Verification items for the finished model (mm, model axes). Face numbers are marked on the shaded views. A direction names the side the tool comes from. Coordinates: 2 decimals unless noted, no trailing zeros. Order: outer loops, then holes, each group sorted by start corner. A loop starts at its lowest first (then second) coordinate and runs counter-clockwise, first axis right, second up. Notation, with made-up numbers: M 69,-32.5 L 100,-32.5 A13 cw 100,-12.5 Z; hole C -3.75,-3 d10. An arc over 180 degrees is marked long. Return JSON: item names as keys, results as strings. Group by question number.
1. Material ranges on line 1 along Y through (x, z) = (-51.75, 5); line 2 along Y through (x, z) = (-42.5, 4.5); line 3 along X through (y, z) = (-14, 4), recorded low to high.
2. Section check D-D, the plane z = 1. Record the cut outline in (x, y).
3. Section check B-B, the plane x = -46.5. Record the cut outline in (y, z), plus the area to 3 significant figures.
4. Set-up check for the marked faces 4 and 5: record each of +Z, -Z, +X, -X, +Y, -Y from which the full face is reachable in a straight line by a thin tool's end or side.
5. Mould release check, pull along X, two halves, no side actions. Record for the marked faces 1, 2 and 3: +X half, -X half, draft (parallel to the pull), parting line (faces both ways), or undercut.
6. Section check A-A, the plane y = -18. Record the cut outline in (x, z).
7. Gauge pin test, flat ends, axial feed: pin 1 (0.8 mm diameter, centred on x = -63.5, z = 4, fed in from -Y); pin 2 (2.5 mm diameter, centred on y = 13.89, z = 5, fed in from -X); pin 3 (2.5 mm diameter, centred on x = -69.5, z = 6, fed in from +Y). Record the tip position at first contact, or that the pin passes through.
8. Section check C-C, the plane y = 17. Record the cut outline in (x, z).
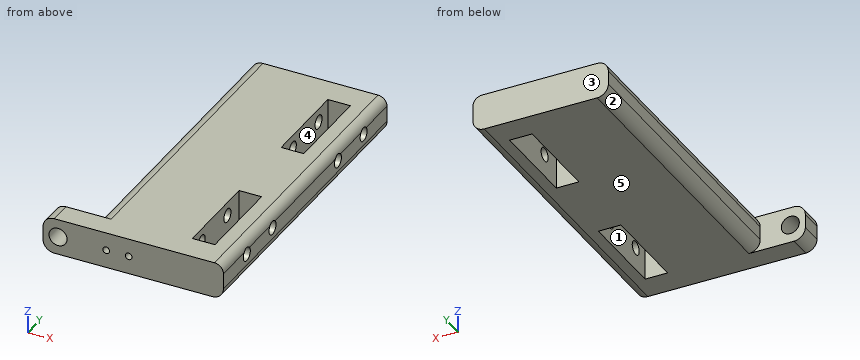
```python
from build123d import *

# Parameters (mm, degrees)
ESBO_O2_W                = 30
ESBO_O2_H                = 70
RESSALTO_EXTRUS_O1_DEPTH = 8
ESBO_O3_R                = 0.75
CORTE_EXTRUS_O1_DEPTH    = 30
FILETE1_R                = 2
ESBO_O17_W               = 10
ESBO_O17_H               = 5
RESSALTO_EXTRUS_O4_DEPTH = 8
ESBO_O20_R               = 2
CORTE_EXTRUS_O9_DEPTH    = 8
FILETE2_R                = 2.5
FILETE3_R                = 2.5
FILETE4_R                = 2.5
FILETE5_R                = 2.5
ESBO_O21_W               = 5
ESBO_O21_H               = 20
CORTE_EXTRUS_O10_DEPTH   = 9
FILETE6_R                = 2.5
ESBO_O22_R               = 1.5
CORTE_EXTRUS_O11_DEPTH   = 20


with BuildPart() as part:
    # Esboço2 → Ressalto-extrusão1 (new body)
    with BuildSketch(Plane.XY):
        with Locations((-52.281248797, -0.107598663)):
            Rectangle(ESBO_O2_W, ESBO_O2_H)
    extrude(amount=RESSALTO_EXTRUS_O1_DEPTH)

    # Esboço3 → Corte-extrusão1 (cut)
    with BuildSketch(Plane(origin=(0, -35.107598663, 0), x_dir=(-1, 0, 0), z_dir=(0, -1, 0))):
        with Locations((58.281248797, -4)):
            Circle(ESBO_O3_R)
        with Locations((63.281248797, -4)):
            Circle(ESBO_O3_R)
    extrude(amount=-CORTE_EXTRUS_O1_DEPTH, mode=Mode.SUBTRACT)

    # Filete1
    filete1_edges = [part.edges().sort_by_distance(p)[0] for p in [
        (-37.281248797, -0.107598663, 8),
    ]]
    fillet(filete1_edges, radius=FILETE1_R)

    # Esboço17 → Ressalto-extrusão4 (add)
    with BuildSketch(Plane(origin=(0, 0, 0), x_dir=(-1, 0, 0), z_dir=(0, 0, -1))):
        with Locations((72.281248797, -32.607598663)):
            Rectangle(ESBO_O17_W, ESBO_O17_H)
    extrude(amount=-RESSALTO_EXTRUS_O4_DEPTH)

    # Esboço20 → Corte-extrusão9 (cut)
    with BuildSketch(Plane.XZ.offset(35.107598663)):
        with Locations((-73.951248797, 4)):
            Circle(ESBO_O20_R)
    extrude(amount=-CORTE_EXTRUS_O9_DEPTH, mode=Mode.SUBTRACT)

    # Filete2
    filete2_edges = [part.edges().sort_by_distance(p)[0] for p in [
        (-67.281248797, 2.392401337, 8),
    ]]
    fillet(filete2_edges, radius=FILETE2_R)

    # Filete3
    filete3_edges = [part.edges().sort_by_distance(p)[0] for p in [
        (-67.281248797, 2.392401337, 0),
    ]]
    fillet(filete3_edges, radius=FILETE3_R)

    # Filete4
    filete4_edges = [part.edges().sort_by_distance(p)[0] for p in [
        (-77.281248797, -32.607598663, 8),
    ]]
    fillet(filete4_edges, radius=FILETE4_R)

    # Filete5
    filete5_edges = [part.edges().sort_by_distance(p)[0] for p in [
        (-77.281248797, -32.607598663, 0),
    ]]
    fillet(filete5_edges, radius=FILETE5_R)

    # Esboço21 → Corte-extrusão10 (cut, through all)
    with BuildSketch(Plane.XY.offset(8)):
        with Locations((-44.781248797, 18.892401337)):
            Rectangle(ESBO_O21_W, ESBO_O21_H)
        with Locations((-44.781248797, -19.107598663)):
            Rectangle(ESBO_O21_W, ESBO_O21_H)
    extrude(amount=-CORTE_EXTRUS_O10_DEPTH, mode=Mode.SUBTRACT)

    # Filete6
    filete6_edges = [part.edges().sort_by_distance(p)[0] for p in [
        (-37.281248797, -0.107598663, 0),
    ]]
    fillet(filete6_edges, radius=FILETE6_R)

    # Esboço22 → Corte-extrusão11 (cut)
    with BuildSketch(Plane(origin=(-37.281248797, 0, 0), x_dir=(0, 0, -1), z_dir=(1, 0, 0))):
        with Locations((-5, -25.107598663)):
            Circle(ESBO_O22_R)
        with Locations((-5, -14.107598663)):
            Circle(ESBO_O22_R)
        with Locations((-5, 24.892401337)):
            Circle(ESBO_O22_R)
        with Locations((-5, 13.892401337)):
            Circle(ESBO_O22_R)
    extrude(amount=-CORTE_EXTRUS_O11_DEPTH, mode=Mode.SUBTRACT)


solid = part.part
```
Answers follow:
{
 "1": {"line 1": "-35.11 to -26.61, -23.61 to -15.61, -12.61 to 12.39, 15.39 to 23.39, 26.39 to 34.89", "line 2": "-35.11 to -29.11, -9.11 to 8.89, 28.89 to 34.89", "line 3": "-67.28 to -64.03, -62.53 to -59.03, -57.53 to -57.28"},
 "2": {"outline": "M -76.78,-35.11 L -37.78,-35.11 L -37.78,34.89 L -66.78,34.89 L -66.78,-30.11 L -76.78,-30.11 Z; hole M -47.28,-29.11 L -42.28,-29.11 L -42.28,-9.11 L -47.28,-9.11 Z; hole M -47.28,8.89 L -42.28,8.89 L -42.28,28.89 L -47.28,28.89 Z"},
 "3": {"outline": "M -35.11,0 L -29.11,0 L -29.11,8 L -35.11,8 Z; M -9.11,0 L 8.89,0 L 8.89,8 L -9.11,8 Z; M 28.89,0 L 34.89,0 L 34.89,8 L 28.89,8 Z", "area": "240 mm^2"},
 "4": {"face 4": "+Z, -Z", "face 5": "-Z, +X, -X, +Y, -Y"},
 "5": {"face 1": "undercut", "face 2": "-X half", "face 3": "draft"},
 "6": {"outline": "M -67.28,2.5 A2.5 ccw -64.78,0 L -47.28,0 L -47.28,8 L -64.78,8 A2.5 ccw -67.28,5.5 Z; M -42.28,0 L -39.78,0 A2.5 ccw -37.28,2.5 L -37.28,6 A2 ccw -39.28,8 L -42.28,8 Z; hole C -63.28,4 d1.5; hole C -58.28,4 d1.5"},
 "7": {"pin 1": "y = -5.11", "pin 2": "x = -67.28", "pin 3": "y = -30.11"},
 "8": {"outline": "M -67.28,2.5 A2.5 ccw -64.78,0 L -47.28,0 L -47.28,8 L -64.78,8 A2.5 ccw -67.28,5.5 Z; M -42.28,0 L -39.78,0 A2.5 ccw -37.28,2.5 L -37.28,6 A2 ccw -39.28,8 L -42.28,8 Z"}
}
